Could you check a few things on this model? Use its own coordinates, in mm. Round coordinates to 2 decimals unless told otherwise and drop trailing zeros. Loops run counter-clockwise (first coordinate to the right, second up) from the corner with the lowest first, then second, coordinate; pieces in that order, holes last.
from build123d import *

# Parameters (mm, degrees)
SKETCH1_W           = 76.2
SKETCH1_H           = 63.5
SKETCH1_R           = 1.3208
SKETCH1_R_2         = 7
BOSS_EXTRUDE1_DEPTH = 2.54


with BuildPart() as part:
    # Sketch1 → Boss-Extrude1 (new body)
    with BuildSketch(Plane.XY):
        Rectangle(SKETCH1_W, SKETCH1_H)
        with Locations((-28, 19.05)):
            Circle(SKETCH1_R, mode=Mode.SUBTRACT)
        with Locations((28, 19.05)):
            Circle(SKETCH1_R, mode=Mode.SUBTRACT)
        with Locations((-28, -12.95)):
            Circle(SKETCH1_R, mode=Mode.SUBTRACT)
        with Locations((28, -12.95)):
            Circle(SKETCH1_R, mode=Mode.SUBTRACT)
        with Locations((0, 9.05)):
            Circle(SKETCH1_R_2, mode=Mode.SUBTRACT)
    extrude(amount=-BOSS_EXTRUDE1_DEPTH)


solid = part.part
Item 1: If we section it at D-D, the plane y = 9.05: Please give me the cut outline in (x, z).
Results list:
outline: (-38.1, -2.54) - (-7, -2.54) - (-7, 0) - (-38.1, 0) - close; (7, -2.54) - (38.1, -2.54) - (38.1, 0) - (7, 0) - close
Item 2: If we section it at C-C, the plane z = -0.9: Please give me the cut outline in (x, y), then the cut area to 3 significant figures.
Results list:
outline: (-38.1, -31.75) - (38.1, -31.75) - (38.1, 31.75) - (-38.1, 31.75) - close; hole circle Ø2.64 at (-28, -12.95); hole circle Ø2.64 at (-28, 19.05); hole circle Ø14 at (0, 9.05); hole circle Ø2.64 at (28, -12.95); hole circle Ø2.64 at (28, 19.05)
area: 4,660 mm2
Item 3: We'd pull the mould along X, two halves only. Please class faces 1 (the flat face through (-1, 31.75, -1)), 2 (the cylindrical face through (3.23, 2.84, -1.25)), 3 (the flat face through (38.1, 0, -1)): released by +X, released by -X, zero draft, split by the parting line, or undercut.
Results list:
face 1: zero draft
face 2: undercut
face 3: released by +X
Item 4: Will this pin go through, and if not, where does the flat tip stop? pin 1 (2 mm diameter, centred on x = -28, y = 19.05, fed in from +Z).
Results list:
pin 1: passes through
Item 5: If I drill on line 1 along Y through (x, z) = (-28, -1.7); line 2 along Y through (x, z) = (0, -1.5); line 3 along Y through (x, z) = (-1.5, -1.35), over which ranges is the centre line in solid material (lowest first)?
Results list:
line 1: y = -31.75 to -14.27, -11.63 to 17.73, 20.37 to 31.75
line 2: y = -31.75 to 2.05, 16.05 to 31.75
line 3: y = -31.75 to 2.21, 15.89 to 31.75
Item 6: If we section it at A-A, the plane x = 0: Please give me the cut outline in (y, z), then the cut area to 3 significant figures.
Results list:
outline: (-31.75, -2.54) - (2.05, -2.54) - (2.05, 0) - (-31.75, 0) - close; (16.05, -2.54) - (31.75, -2.54) - (31.75, 0) - (16.05, 0) - close
area: 126 mm2
Item 7: If we section it at B-B, the plane y = -12.95: Please give me the cut outline in (x, z), then the cut area to 3 significant figures.
Results list:
outline: (-38.1, -2.54) - (-29.32, -2.54) - (-29.32, 0) - (-38.1, 0) - close; (-26.68, -2.54) - (26.68, -2.54) - (26.68, 0) - (-26.68, 0) - close; (29.32, -2.54) - (38.1, -2.54) - (38.1, 0) - (29.32, 0) - close
area: 180 mm2
